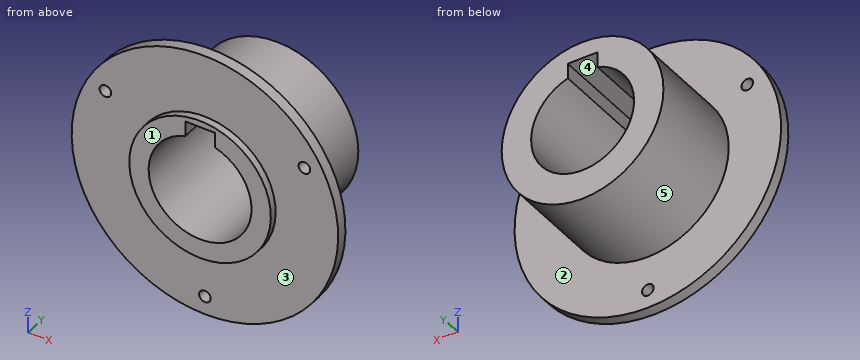
from build123d import *

# Parameters (mm, degrees)
F_1_8_0_125_DIAMETER_HOLE1_D = 3.175
CIRPATTERN1_COUNT            = 3
CUT_EXTRUDE2_DEPTH           = 61.432813934


with BuildPart() as part:
    # Sketch1 → Revolve1 (revolve)
    with BuildSketch(Plane.XY, mode=Mode.PRIVATE) as revolve1_sk:
        Polygon((22, 30), (22, 3), (36.25, 3), (36.25, 0), (19.25, 0), (19.25, -2), (14, -2), (14, 30), align=None)
    revolve(revolve1_sk.sketch.rotate(Axis((0, 0, 0), (0, 1, 0)), 90), axis=Axis((0, 0, 0), (0, 1, 0)))

    # 1/8 (0.125) Diameter Hole1 (through all)
    with Locations(Plane(origin=(0, 3, 0), x_dir=(1, 0, 0), z_dir=(0, 1, 0))):
        with Locations((0, 31.25)):
            f_1_8_0_125_diameter_hole1 = Hole(F_1_8_0_125_DIAMETER_HOLE1_D / 2)

    # CirPattern1: 1/8 (0.125) Diameter Hole1 ×3 about axis
    cirpattern1_axis = Axis((0, 0, 0), (0, 1, 0))
    for i in range(1, CIRPATTERN1_COUNT):
        add(f_1_8_0_125_diameter_hole1.rotate(cirpattern1_axis, i * 360 / CIRPATTERN1_COUNT), mode=Mode.SUBTRACT)

    # Sketch7 → Cut-Extrude2 (cut, through all)
    with BuildSketch(Plane(origin=(0, 30, 0), x_dir=(1, 0, 0), z_dir=(0, 1, 0))):
        Polygon((0, -17.5), (4, -17.5), (4, -12.919453698), (-4, -12.919453698), (-4, -17.5), align=None)
    extrude(amount=-CUT_EXTRUDE2_DEPTH, mode=Mode.SUBTRACT)


solid = part.part
Here's how the part is built. I have some questions about the finished solid (model axes, mm). Face numbers are marked on the shaded views. A direction names the side the tool comes from. Coordinates: 2 decimals unless noted, no trailing zeros. Order: outer loops, then holes, each group sorted by start corner. A loop starts at its lowest first (then second) coordinate and runs counter-clockwise, first axis right, second up. Notation, with made-up numbers: M 22.5,60 L 72.5,60 A20 ccw 72.5,64 Z; hole C 50,58 d8. An arc over 180 degrees is marked long. Answer as CSV lines item,"result". Start each with the question number.
1. For pin 1 (4 mm diameter, centred on x = 27.06, z = 15.63, fed in from -Y); pin 2 (8 mm diameter, centred on y = 20.5, z = -13, fed in from +X); pin 3 (4 mm diameter, centred on x = 17, z = 19.5, fed in from +Y), each with a flat end and sliding along its axis, tell me the tip position at first contact or that it passes through.
2. I want a section at A-A, the plane z = 0. Write out the boundary of the cut face in (x, y), and give its area (4 significant figures).
3. On a 3-axis mill with a long thin cutter (end or side, diameter ignored), from which of +Z, -Z, +X, -X, +Y, -Y can I reach the whole of each face in a straight line? I mean the marked faces 1 and 2. Say none if no direction works.
4. I want a section at C-C, the plane y = 23. Write out the boundary of the cut face in (x, z).
5. I want a section at D-D, the plane y = 2. Count the separate pieces of the cut face and the enclosed holes in it, and give its area (3 significant figures).
6. I want a section at B-B, the plane x = 0. Write out the boundary of the cut face in (y, z).
7. We'd pull the mould along Z, two halves only. Please class the marked faces 3, 4 and 5: released by +Z, released by -Z, zero draft, split by the parting line, or undercut.
8. I need wall thicknesses on line 1 (Y direction, x = 16, z = -12.5); line 2 (Y direction, x = 24.5, z = 0.5); line 3 (X direction, y = 2, z = 4.5). Which ranges of each line are inside material? Lowest first, please. Write a range as [from, to].
Recorded:
1,pin 1,"stops at y = 0"
1,pin 2,"stops at x = 20.07"
1,pin 3,"stops at y = 3"
2,outline,"M -36.25,0 L -19.25,0 L -19.25,-2 L -14,-2 L -14,30 L -22,30 L -22,3 L -36.25,3 Z; M 14,-2 L 19.25,-2 L 19.25,0 L 36.25,0 L 36.25,3 L 22,3 L 22,30 L 14,30 Z"
2,area,"586.5 mm2"
3,face 1,"+Z, -Z, +X, -X, -Y"
3,face 2,"+Y"
4,outline,"C 0,0 d44; hole M -4,13.42 A14 ccw long 4,13.42 L 4,17.5 L -4,17.5 Z"
5,separate pieces,"1"
5,enclosed holes,"4"
5,area,"3,460 mm2"
6,outline,"M -2,-19.25 L 0,-19.25 L 0,-29.66 L 3,-29.66 L 3,-22 L 30,-22 L 30,-14 L -2,-14 Z; M -2,17.5 L 30,17.5 L 30,22 L 3,22 L 3,36.25 L 0,36.25 L 0,19.25 L -2,19.25 Z; M 0,-36.25 L 3,-36.25 L 3,-32.84 L 0,-32.84 Z"
7,face 3,"zero draft"
7,face 4,"undercut"
7,face 5,"split by the parting line"
8,line 1,"y = [0, 30]"
8,line 2,"y = [0, 3]"
8,line 3,"x = [-35.97, -13.26], [13.26, 35.97]"
